Source: three-view drawing plus pictorial views. Frame: mm from the lowest corner of the part. Coordinates: 2 decimals unless noted, no trailing zeros. Loops run counter-clockwise (first coordinate to the right, second up) from the corner with the lowest first, then second, coordinate; pieces in that order, holes last. Notation, with made-up numbers: M 15,33.25 L 52,33.25 A23 cw 52,65.25 Z; hole C 11.25,-17 d6. An arc over 180 degrees is marked long. Use a Markdown table: item, result. Add a question column.
1. Section C-C on y = 1.05. Output: boundary loops of the cut face in (x, z), then the cut area to 3 significant figures.
2. Line query: L1, parallel to X at y = 0.8, z = 26; L2, parallel to Z at x = 5, y = 1.1; L3, parallel to X at y = 1.25, z = 15.5. Output: solid intervals per line, ascending. Write a range as [from, to].
3. Section A-A on z = 27. Output: boundary loops of the cut face in (x, y).
4. Section D-D on z = 15.5. Output: boundary loops of the cut face in (x, y).
5. Pin query (flat end, axial travel): pin 1 (12 mm diameter, centred on x = 21.5, z = 17, fed in from -Y). Return the tip coordinate at first contact, or that it passes through.
6. Section B-B on x = 5. Output: boundary loops of the cut face in (y, z).
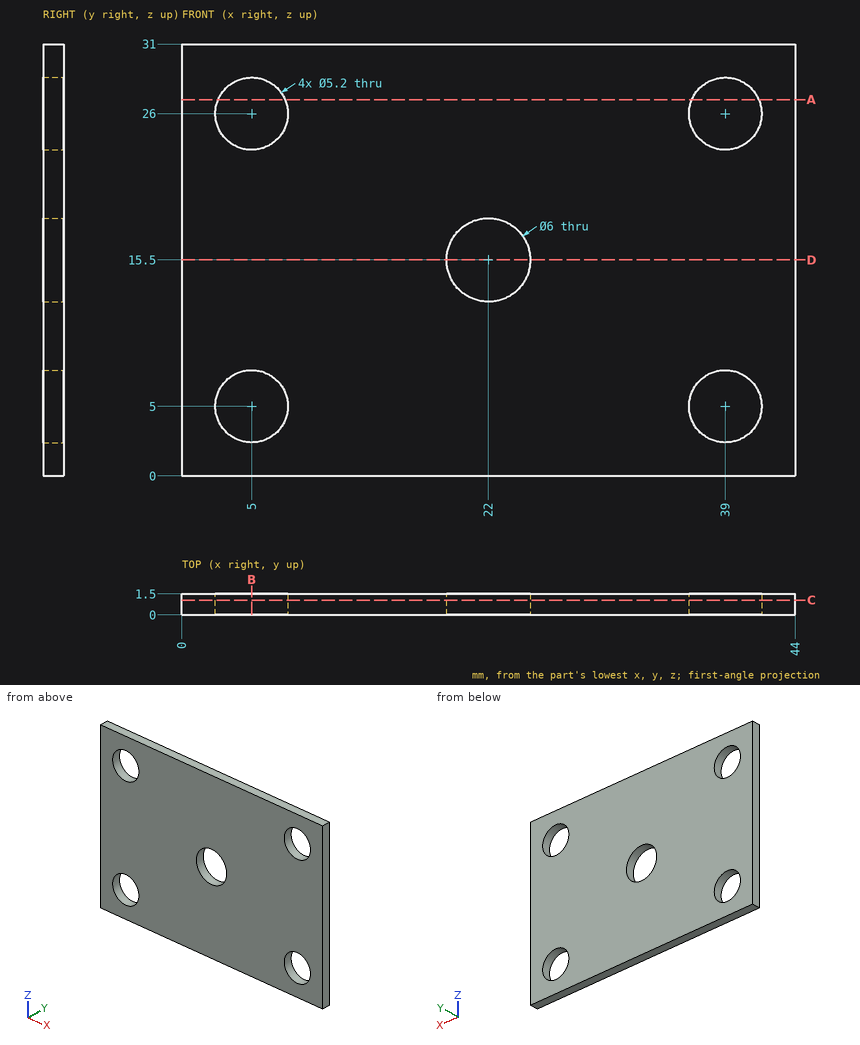
Answers below:
| question | item | result |
|---|---|---|
| 1 | outline | M 0,0 L 44,0 L 44,31 L 0,31 Z; hole C 5,5 d5.2; hole C 5,26 d5.2; hole C 22,15.5 d6; hole C 39,5 d5.2; hole C 39,26 d5.2 |
| 1 | area | 1,250 mm² |
| 2 | L1 | x = [0, 2.4], [7.6, 36.4], [41.6, 44] |
| 2 | L2 | z = [0, 2.4], [7.6, 23.4], [28.6, 31] |
| 2 | L3 | x = [0, 19], [25, 44] |
| 3 | outline | M 0,0 L 2.6,0 L 2.6,1.5 L 0,1.5 Z; M 7.4,0 L 36.6,0 L 36.6,1.5 L 7.4,1.5 Z; M 41.4,0 L 44,0 L 44,1.5 L 41.4,1.5 Z |
| 4 | outline | M 0,0 L 19,0 L 19,1.5 L 0,1.5 Z; M 25,0 L 44,0 L 44,1.5 L 25,1.5 Z |
| 5 | pin 1 | stops at y = 0 |
| 6 | outline | M 0,0 L 1.5,0 L 1.5,2.4 L 0,2.4 Z; M 0,7.6 L 1.5,7.6 L 1.5,23.4 L 0,23.4 Z; M 0,28.6 L 1.5,28.6 L 1.5,31 L 0,31 Z |
